For this review, use the dimensioned drawing (mm, ordinates from the lowest corner) and the shaded views. A direction names the side the tool comes from. Coordinates: 2 decimals unless noted, no trailing zeros. Loops run counter-clockwise (first coordinate to the right, second up) from the corner with the lowest first, then second, coordinate; pieces in that order, holes last. Notation, with made-up numbers: (27.5, 74.25) -> (60.5, 74.25) arc R20 cw to (60.5, 99.25) -> close; hole circle Ø11 at (30, 27.5). An arc over 180 degrees is marked (long way). Answer as a JSON object with one key per item and string values.
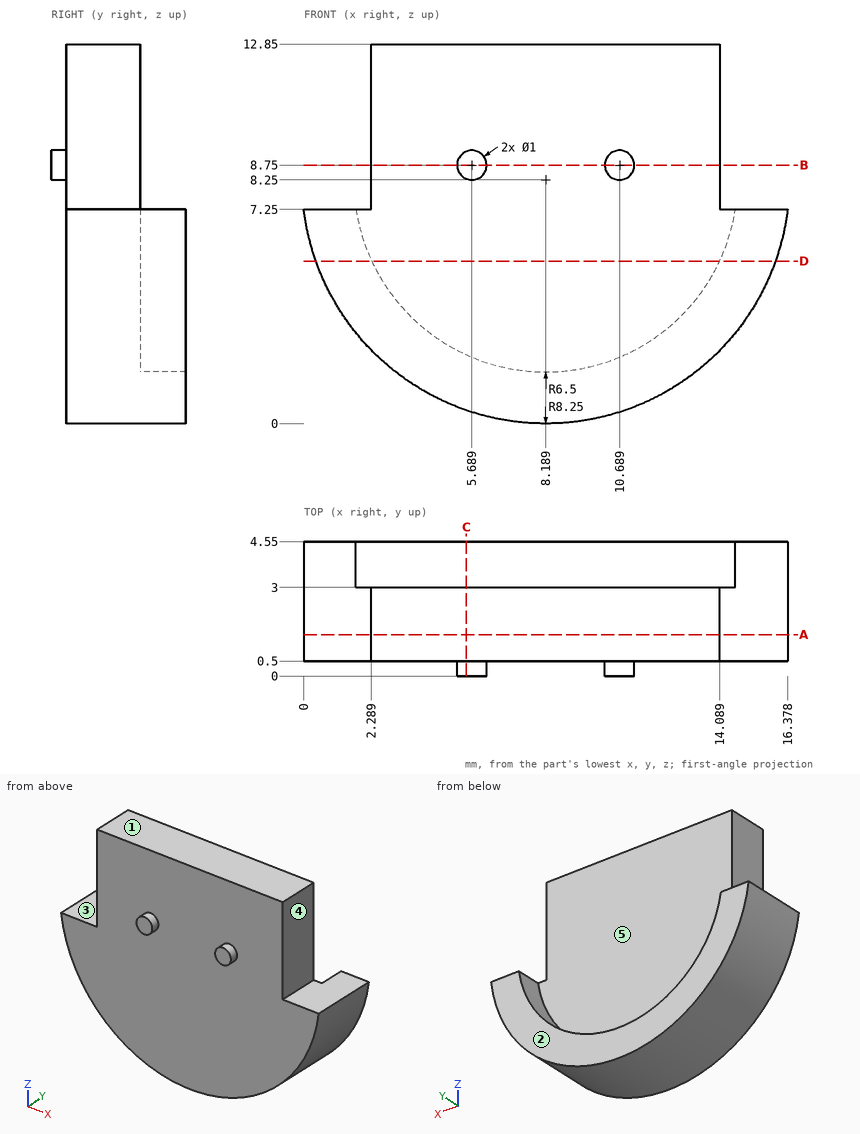
1) Add section C-C, the plane x = 5.5. Give the boundary of the cut face in (y, z), and give its area (3 significant figures).
Completed:
{"outline": "(0, 8.29) -> (0.5, 8.29) -> (0.5, 0.45) -> (4.55, 0.45) -> (4.55, 2.33) -> (3, 2.33) -> (3, 12.85) -> (0.5, 12.85) -> (0.5, 9.21) -> (0, 9.21) -> close", "area": "34.4 mm²"}
2) Wall thickness on probe 1 along Y at (x, z) = (6.5, 6); probe 2 along Y at (x, z) = (12, 1.5); probe 3 along X at (y, z) = (2.45, 11.75): over which ranges is each line inside the solid? List them lowest first.
Completed:
{"probe 1": "0.5 to 3", "probe 2": "0.5 to 4.55", "probe 3": "2.29 to 14.09"}
3) Add section A-A, the plane y = 1.4. Give the boundary of the cut face in (x, z).
Completed:
{"outline": "(0, 7.25) arc R8.25 ccw to (16.38, 7.25) -> (14.09, 7.25) -> (14.09, 12.85) -> (2.29, 12.85) -> (2.29, 7.25) -> close"}
4) Clearance check with flat-ended pins moving along their axes: pin 1 Ø2 at (y, z) = (2, 9.5) entering from +X; pin 2 Ø1.2 at (y, z) = (2, 9) entering from -X; pin 3 Ø3.5 at (x, z) = (11, 7) entering from +Y. State where each tip first meets the part, or that it passes through.
Completed:
{"pin 1": "x = 14.09", "pin 2": "x = 2.29", "pin 3": "y = 3"}
5) For the marked faces 1, 2, 3, 4 and 5, list the 3-axis set-ups (+Z, -Z, +X, -X, +Y, -Y) from which the entire face can be reached by the end or side of a thin tool; tool diameter is ignored.
Completed:
{"face 1": "+Z, +X, -X, +Y, -Y", "face 2": "+Z, -Z, +X, -X, +Y", "face 3": "+Z, -X, +Y, -Y", "face 4": "+Z, +X, +Y, -Y", "face 5": "+Z, +Y"}
6) Add section B-B, the plane z = 8.75. Give the boundary of the cut face in (x, y), and give its area (3 significant figures).
Completed:
{"outline": "(2.29, 0.5) -> (5.19, 0.5) -> (5.19, 0) -> (6.19, 0) -> (6.19, 0.5) -> (10.19, 0.5) -> (10.19, 0) -> (11.19, 0) -> (11.19, 0.5) -> (14.09, 0.5) -> (14.09, 3) -> (2.29, 3) -> close", "area": "30.5 mm²"}
7) Add section D-D, the plane z = 5.5. Give the boundary of the cut face in (x, y).
Completed:
{"outline": "(0.41, 0.5) -> (15.97, 0.5) -> (15.97, 4.55) -> (14.08, 4.55) -> (14.08, 3) -> (2.3, 3) -> (2.3, 4.55) -> (0.41, 4.55) -> close"}
